Geometry check sheet. Reference: drawing and pictorial views, mm from the part's lowest x, y, z. Give positions to 0.01 mm unless a question says otherwise; leave off trailing zeros. Loops run counter-clockwise (first coordinate to the right, second up) from the corner with the lowest first, then second, coordinate; pieces in that order, holes last. Notation, with made-up numbers: (75, 27.5) - (83, 27.5) arc R13 cw to (83, 39.5) - close; hole circle Ø10 at (29, -14). An arc over 180 degrees is marked (long way). Answer in a Markdown table with one row per item. Add a question column.
(1) Sectioned sample at A-A on x = 228.5. Enter the section's corners in (y, z), then the cut area to 3 significant figures.
(2) Sectioned sample at B-B on z = 458. Enter the section's corners in (x, y).
(3) Thickness scan on L1, parallel to X at y = 12, z = 50; L2, parallel to Z at x = 228.5, y = 14; L3, parallel to Z at x = 226.5, y = 31.5. Record the ranges inside material, lowest first.
(4) Go/stop test with flat-tipped pins: P1, Ø8, axis at x = 214, y = 82.5, coming from the -Z side; P2, Ø20, axis at x = 222.5, z = 453.5, coming from the -Y side. Record where each tip stops, or that it passes through.
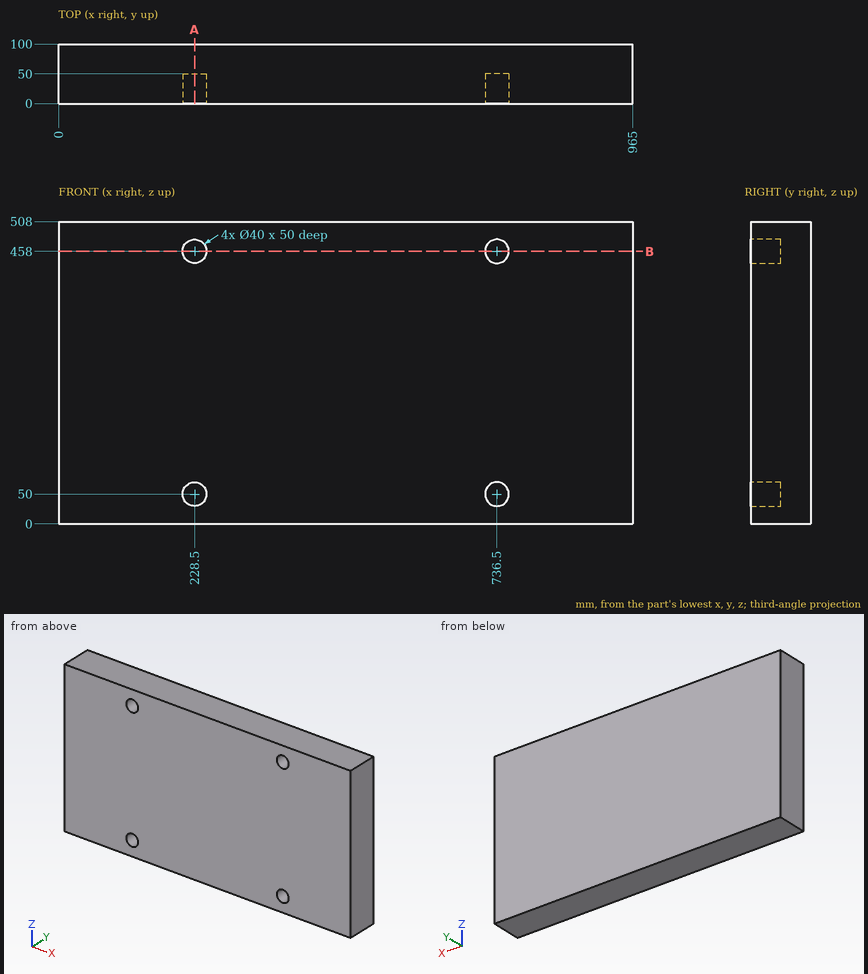
Reply:
| question | item | result |
|---|---|---|
| 1 | outline | (0, 0) - (100, 0) - (100, 508) - (0, 508) - (0, 478) - (50, 478) - (50, 438) - (0, 438) - (0, 70) - (50, 70) - (50, 30) - (0, 30) - close |
| 1 | area | 46,800 mm^2 |
| 2 | outline | (0, 0) - (208.5, 0) - (208.5, 50) - (248.5, 50) - (248.5, 0) - (716.5, 0) - (716.5, 50) - (756.5, 50) - (756.5, 0) - (965, 0) - (965, 100) - (0, 100) - close |
| 3 | L1 | 0 to 208.5, 248.5 to 716.5, 756.5 to 965 |
| 3 | L2 | 0 to 30, 70 to 438, 478 to 508 |
| 3 | L3 | 0 to 30.1, 69.9 to 438.1, 477.9 to 508 |
| 4 | P1 | z = 0 |
| 4 | P2 | y = 50 |
